Autodesk Inventor part; units mm, degrees
ref_plane "YZ Plane" through (0, 0, 0) normal (1, 0, 0) x (0, 1, 0)
ref_plane "XZ Plane" through (0, 0, 0) normal (0, 1, 0) x (-1, 0, 0)
ref_plane "XY Plane" through (0, 0, 0) normal (0, 0, 1) x (1, 0, 0)
sketch "Sketch1" plane through (0, 0, 0) normal (0, 0, 1) x (1, 0, 0)
  circle A0 centre (0, 0) radius 25
  dimension "d0" = 50
extrude "Extrusion1" add sketch "Sketch1" along normal mid plane 50
sketch "Sketch2" plane through (0, 0, 0) normal (1, 0, 0) x (0, 1, 0)
  circle A0 centre (0, 0) radius 20
  line L0 (25, 25) -> (-25, 25)
  line L1 (-25, -25) -> (25, -25)
  line L2 (25, 25) -> (21, 25)
  line L3 (21, 25) -> (21, -25)
  line L4 (21, -25) -> (25, -25)
  line L5 (25, -25) -> (25, 25)
  dimension "d3" = 40
  dimension "d4" = 4
extrude "Extrusion2" add sketch "Sketch2" along normal blind 85
sketch "Sketch3" plane through (0, 0, 0) normal (0, 0, 1) x (1, 0, 0)
  circle A0 centre (0, 0) radius 12.5
  dimension "d7" = 25
extrude "Extrusion3" cut sketch "Sketch3" along normal through all both and the other way through all
sketch "Sketch4" plane through (85, 0, 0) normal (1, 0, 0) x (0, 0, -1)
  circle A0 centre (0, 0) radius 17.5
  dimension "d10" = 35
extrude "Extrusion4" add sketch "Sketch4" along normal blind 2
sketch "Sketch5" plane through (87, 0, 0) normal (1, 0, 0) x (0, 0, -1)
  circle A0 centre (0, 0) radius 10
  dimension "d13" = 20
extrude "Extrusion5" add sketch "Sketch5" along normal blind 35
sketch "Sketch6" plane through (122, 0, 0) normal (1, 0, 0) x (0, 0, -1)
  circle A0 centre (0, 0) radius 7.5
  dimension "d16" = 15
extrude "Extrusion6" add sketch "Sketch6" along normal blind 45
sketch "Sketch7" plane through (0, 0, 0) normal (0, 0, 1) x (1, 0, 0)
  circle A0 centre (157, 0) radius 3.75
  line L0 (167, -7.5) -> (167, 7.5)
  point P0 (0, 0)
  dimension "d19" = 7.5
  dimension "d20" = 10
extrude "Extrusion7" cut sketch "Sketch7" along normal through all both and the other way through all
chamfer "Chamfer1" distance 0.5 angle 45 2 edges at (85, -20, 0) (87, 0, 17.5)
chamfer "Chamfer2" distance 1 angle 45 1 edges at (122, 0, 10)
fillet "Fillet1" radius 5 1 edges at (167, 0, 7.5)
sketch "Sketch8" plane through (0, 0, 0) normal (0, 0, 1) x (1, 0, 0)
  arc A0 (-12.5, 0) -> (0, -12.5) centre (0, 0) ccw
  arc A1 (-25, 0) -> (0, -25) centre (0, 0) ccw
  line L0 (0, 0) -> (-25, 0)
  line L1 (0, 0) -> (0, -25)
  dimension "d30" = 25
  dimension "d31" = 50
extrude "Extrusion8" cut sketch "Sketch8" along normal mid plane 15 contours A0 L1 A1 L0
sketch "Sketch9" plane through (0, 0, 0) normal (0, 1, 0) x (-1, 0, 0)
  line L0 (-167, -2.5) -> (-167, 2.5)
  line L1 (-167, -2.5) -> (-147, -2.5)
  line L2 (-147, -2.5) -> (-147, 2.5)
  line L3 (-147, 2.5) -> (-167, 2.5)
  point P0 (0, 0)
  dimension "d34" = 20
extrude "Extrusion9" cut sketch "Sketch9" along normal through all both and the other way through all
properties part number "Hydraulic Arm"
Read the model definition and answer for the solid it produces. Units are mm, in the model's axes. A direction names the side the tool comes from. Give positions to 0.01 mm unless a question says otherwise; leave off trailing zeros. Order: outer loops, then holes, each group sorted by start corner. A loop starts at its lowest first (then second) coordinate and runs counter-clockwise, first axis right, second up.
(1) Straight lines are drawn through the part: L1, parallel to Y at x = 48, z = 4.5; L2, parallel to Y at x = 0, z = 8; L3, parallel to Y at x = 111.5, z = 0. For each, find the intervals that lie inside material, in ascending order.
(2) For faces 1 (the flat face through (159.4, -3.2, -2.5)), 2 (the flat face through (-13, -12, 7.5)), 3 (the flat face through (122, 7.4, 2)), determine the directions among +Z, -Z, +X, -X, +Y, -Y from which every point of the face is accessible in a straight line to the end or side of a thin tool.
(3) Given pin 1 (15.5 mm diameter, centred on x = 153, y = 2.5, fed in from +Z); pin 2 (7 mm diameter, centred on x = 156.5, y = 0.5, fed in from -Z); pin 3 (12 mm diameter, centred on x = 56.5, z = -9.5, fed in from -Y); pin 4 (15 mm diameter, centred on x = 0, y = 0, fed in from -Z), each flat-ended and moving along its own axis, determine where each tip first touches the part or whether it passes through.
(4) Find section D-D (x = 157). Give the vertices of the cut face in (y, z).
(5) Find section C-C (x = 67.5). Give the vertices of the cut face in (y, z), plus the area to 3 significant figures.
(6) For a pull along Y with two mould halves and no side action, classify faces 4 (the flat face through (154.6, -3.2, 2.5)), 5 (the cylindrical face through (49.263, 18.475, 7.66)), 6 (the cylindrical face through (137.276, 6.654, -3.461)), 7 (the cylindrical face through (160.464, -1.436, 5.035)) as released by +Y, released by -Y, zero draft, split by the parting line, or undercut.
(7) Find section B-B (x = -9). Give the vertices of the cut face in (y, z), plus the area to 3 significant figures.
Result sheet:
1. L1: y = -19.49 to 19.49, 21 to 25
1. L2: y = -25 to -12.5, 12.5 to 25
1. L3: y = -10 to 10
2. face 1: +X, +Y, -Y
2. face 2: -X, -Y
2. face 3: +X
3. pin 1: stops at z = 7.5
3. pin 2: stops at z = -7.5
3. pin 3: stops at y = -19.69
3. pin 4: passes through
4. outline: (-7.07, -2.5) arc R7.5 ccw to (-3.75, -6.5) - (-3.75, -2.5) - close; (-7.07, 2.5) - (-3.75, 2.5) - (-3.75, 6.5) arc R7.5 ccw to start; (3.75, -6.5) arc R7.5 ccw to (7.07, -2.5) - (3.75, -2.5) - close; (3.75, 2.5) - (7.07, 2.5) arc R7.5 ccw to (3.75, 6.5) - close
5. outline: circle Ø40 at (0, 0); (21, -25) - (25, -25) - (25, 25) - (21, 25) - close
5. area: 1,460 mm2
6. face 4: zero draft
6. face 5: undercut
6. face 6: split by the parting line
6. face 7: undercut
7. outline: (-23.32, -25) - (-8.67, -25) - (-8.67, -7.5) - (-23.32, -7.5) - close; (-23.32, 7.5) - (-8.67, 7.5) - (-8.67, 25) - (-23.32, 25) - close; (8.67, -25) - (23.32, -25) - (23.32, 25) - (8.67, 25) - close
7. area: 1,250 mm2
